Drawing for the job (mm, zero at the part's lowest x, y, z). A direction names the side the tool comes from. Round coordinates to 2 decimals unless told otherwise and drop trailing zeros. Order: outer loops, then holes, each group sorted by start corner. A loop starts at its lowest first (then second) coordinate and runs counter-clockwise, first axis right, second up. Notation, with made-up numbers: (24.25, 38.5) - (34.25, 38.5) arc R14 ccw to (34.25, 57.5) - close; hole circle Ø9 at (63, 60). An arc over 180 degrees is marked (long way). Put each result on its own line as item: value. Start each with the question number.
Item 1: Saw through at A-A on x = 2.65. List the corners of the cut face in (y, z).
Item 2: Saw through at C-C on y = 0.45. List the corners of the cut face in (x, z).
Item 3: Which spindle directions (+Z, -Z, +X, -X, +Y, -Y) get a long thin tool onto all of the face, cutting with end or side? Do the marked faces 1, 2, 3 and 4. Say none if no direction does.
Item 4: Saw through at D-D on x = 0.65. List the corners of the cut face in (y, z).
Item 5: Probe probe 1 along X at (y, z) = (0.7, 2); probe 2 along Y at (x, z) = (0.4, 2.3); probe 3 along Z at (x, y) = (2.9, 3.75). List the from-to ranges inside material, lowest first.
Item 6: Pin check, flat tips, straight feed: pin 1 Ø0.5 at (x, y) = (2, 4.5) entering from -Z; pin 2 Ø2 at (x, y) = (2.5, 2.5) entering from -Z. Stop position of each tip, or through.
Item 7: Mould opens along Y. For the marked faces 5, 6 and 7 say: pulls with the +Y half, pulls with the -Y half, needs draft (parallel to the pull), parting line crosses it, or undercut.
Item 8: Saw through at B-B on z = 3.35. List the corners of the cut face in (x, y).
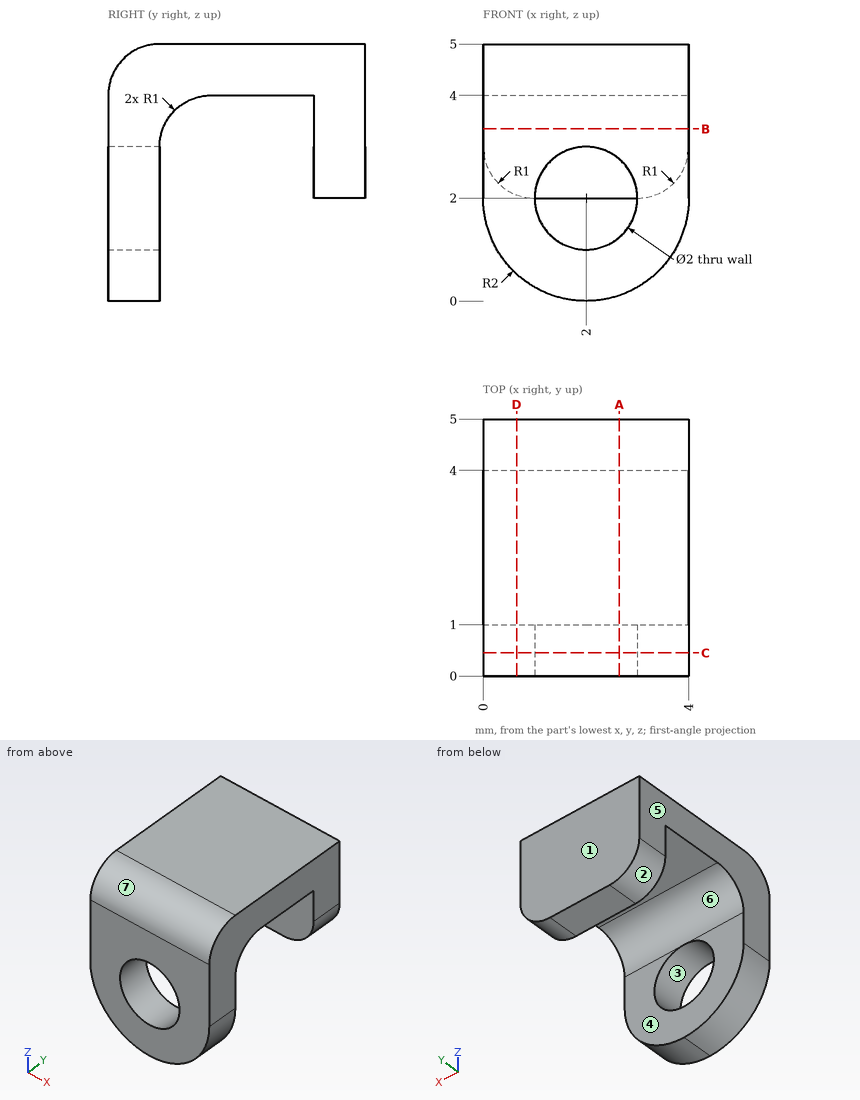
Results found:
1. outline: (0, 0.11) - (1, 0.11) - (1, 1.24) - (0, 1.24) - close; (0, 2.76) - (1, 2.76) - (1, 3) arc R1 cw to (2, 4) - (4, 4) - (4, 2) - (5, 2) - (5, 5) - (1, 5) arc R1 ccw to (0, 4) - close
2. outline: (0, 2) arc R2 ccw to (4, 2) - (4, 4.84) - (0, 4.84) - close; hole circle Ø2 at (2, 2)
3. face 1: +Z, -Z, +X, -X, +Y
3. face 2: -Z, -X, +Y
3. face 3: -Y
3. face 4: -Z, +X, -X
4. outline: (0, 0.52) - (1, 0.52) - (1, 3) arc R1 cw to (2, 4) - (4, 4) - (4, 2.06) - (5, 2.06) - (5, 5) - (1, 5) arc R1 ccw to (0, 4) - close
5. probe 1: x = 0 to 1, 3 to 4
5. probe 2: y = 0 to 1, 4 to 5
5. probe 3: z = 4 to 5
6. pin 1: stops at z = 2
6. pin 2: stops at z = 3.87
7. face 5: needs draft
7. face 6: undercut
7. face 7: pulls with the -Y half
8. outline: (0, 0) - (4, 0) - (4, 1.06) - (0, 1.06) - close; (0, 4) - (4, 4) - (4, 5) - (0, 5) - close
